Input: part model. Units: mm. Frame: model coordinates. Coordinates: 2 decimals unless noted, no trailing zeros. Write each loop counter-clockwise with the first axis right and the second up, starting at its lowest first coordinate (ties: lowest second). Pieces come first, ordered by that corner, then holes. Notation, with made-up numbers: M 50.5,-26.5 L 90.5,-26.5 A24 ccw 90.5,-5.5 Z; hole C 7,38 d7. An arc over 180 degrees is marked long. Answer as a JSON object with one key per item and string values. Group by question number.
Autodesk Fusion 360 part; units mm, degrees
sketch "Sketch1" plane through (0, 0, 0) normal (0, 0, 1) x (1, 0, 0)
  circle A0 centre (0, 0) radius 7.5
  line L0 (2.2175, 7.1647) -> (7.4999, -0.0289)
  dimension "d1" = 15
extrude "Extrude1" add sketch "Sketch1" along normal blind 400 contours A0 L0 picked at (-0.1624, -2.0405)
chamfer "Chamfer1" distance 0.5 angle 45 1 faces at (7.461, -0.7641, 133.3333)
sketch "Sketch2" plane through (0, 0, 400) normal (0, 0, 1) x (-1, 0, 0)
  arc A0 (-2.7525, -6.4361) -> (-6.9649, -0.6997) centre (0, 0) ccw
  line L0 (-6.9649, -0.6997) -> (-2.7525, -6.4361)
Q1. Section A-A, the plane z = 96. Return the cut outline in (x, y), and give its area (3 significant figures).
Q2. Pin query (flat end, axial travel): pin 1 Ø5 at (x, z) = (-3, 279) entering from -Y; pin 2 Ø3 at (y, z) = (5, 89.5) entering from -X. Return the tip coordinate at first contact, or that it passes through.
Q3. Line query: line 1 (Y direction, x = 0.75, z = 238); line 2 (X direction, y = -0.5, z = 77); line 3 (Z direction, x = -6.75, y = -2.75). Output: solid intervals per line, ascending. Write a range as from..to.
Filled in:
{
 "1": {"outline": "M 1.74,7.3 A7.5 ccw long 7.48,-0.53 L 7.2,0.37 L 2.51,6.76 Z", "area": "168 mm^2"},
 "2": {"pin 1": "y = -7.48", "pin 2": "x = -6.63"},
 "3": {"line 1": "-7.46..7.46", "line 2": "-7.48..7.47", "line 3": "0.29..399.71"}
}
